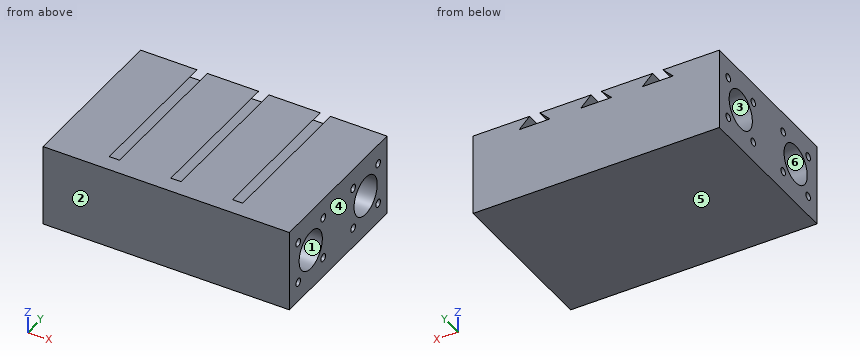
from build123d import *

# Parameters (mm, degrees)
SKETCH1_W                        = 120
SKETCH1_H                        = 80
BOSS_EXTRUDE1_DEPTH              = 40
SKETCH2_R                        = 1.85
LINEAR_BEARING_SCREW_CUTS_DEPTH  = 14
SKETCH3_R                        = 9.5
LINEAR_BEARINGS_HOLE_DEPTH       = 55
SKETCH4_R                        = 1.875
LINEAR_BEARING_SCREW_CUTS2_DEPTH = 14
LINEAR_BEARINGS_HOLE2_START      = -55
SKETCH5_R                        = 9.5
LINEAR_BEARINGS_HOLE2_DEPTH      = 55
CUT_EXTRUDE7_DEPTH               = 72


with BuildPart() as part:
    # Sketch1 → Boss-Extrude1 (new body)
    with BuildSketch(Plane.XY):
        with Locations((60, 40)):
            Rectangle(SKETCH1_W, SKETCH1_H)
    extrude(amount=BOSS_EXTRUDE1_DEPTH)

    # Sketch2 → linear-bearing-screw-cuts (cut)
    with BuildSketch(Plane.ZY):
        with Locations((30.25, 72.75)):
            Circle(SKETCH2_R)
        with Locations(Location((9.75, 72.75, 0), (0, 0, 180))):
            Circle(SKETCH2_R)
        with Locations(Location((30.25, 52.25, 0), (0, 0, 180))):
            Circle(SKETCH2_R)
        with Locations((9.75, 52.25)):
            Circle(SKETCH2_R)
        with Locations(Location((9.75, 27.75, 0), (0, 0, 180))):
            Circle(SKETCH2_R)
        with Locations((30.25, 27.75)):
            Circle(SKETCH2_R)
        with Locations(Location((30.25, 7.25, 0), (0, 0, 180))):
            Circle(SKETCH2_R)
        with Locations((9.75, 7.25)):
            Circle(SKETCH2_R)
    extrude(amount=-LINEAR_BEARING_SCREW_CUTS_DEPTH, mode=Mode.SUBTRACT)

    # Sketch3 → linear-bearings-hole (cut)
    with BuildSketch(Plane.ZY):
        with Locations((20, 62.5)):
            Circle(SKETCH3_R)
        with Locations(Location((20, 17.5, 0), (0, 0, 180))):
            Circle(SKETCH3_R)
    extrude(amount=-LINEAR_BEARINGS_HOLE_DEPTH, mode=Mode.SUBTRACT)

    # Sketch4 → linear-bearing-screw-cuts2 (cut)
    with BuildSketch(Plane(origin=(120, 0, 0), x_dir=(0, 0, -1), z_dir=(1, 0, 0))):
        with Locations((-9.75, 72.75)):
            Circle(SKETCH4_R)
        with Locations(Location((-30.25, 72.75, 0), (0, 0, 180))):
            Circle(SKETCH4_R)
        with Locations(Location((-9.75, 52.25, 0), (0, 0, 180))):
            Circle(SKETCH4_R)
        with Locations((-30.25, 52.25)):
            Circle(SKETCH4_R)
        with Locations(Location((-30.25, 27.75, 0), (0, 0, 180))):
            Circle(SKETCH4_R)
        with Locations((-9.75, 27.75)):
            Circle(SKETCH4_R)
        with Locations(Location((-9.75, 7.25, 0), (0, 0, 180))):
            Circle(SKETCH4_R)
        with Locations((-30.25, 7.25)):
            Circle(SKETCH4_R)
    extrude(amount=-LINEAR_BEARING_SCREW_CUTS2_DEPTH, mode=Mode.SUBTRACT)

    # Sketch5 → linear-bearings-hole2 (cut)
    with BuildSketch(Plane(origin=(120, 0, 0), x_dir=(0, 0, -1), z_dir=(1, 0, 0)).offset(LINEAR_BEARINGS_HOLE2_START)):
        with Locations(Location((-20, 62.5, 0), (0, 0, 180))):
            Circle(SKETCH5_R)
        with Locations((-20, 17.5)):
            Circle(SKETCH5_R)
    extrude(amount=LINEAR_BEARINGS_HOLE2_DEPTH, mode=Mode.SUBTRACT)

    # Sketch10 → Cut-Extrude7 (cut)
    with BuildSketch(Plane(origin=(0, 80, 0), x_dir=(1, 0, 0), z_dir=(0, 1, 0))):
        Polygon((92.5, -40), (97.5, -35), (82.5, -35), (87.5, -40), align=None)
        Polygon((67.5, -35), (62.5, -40), (57.5, -40), (52.5, -35), align=None)
        Polygon((37.5, -35), (32.5, -40), (27.5, -40), (22.5, -35), align=None)
    extrude(amount=-CUT_EXTRUDE7_DEPTH, mode=Mode.SUBTRACT)


solid = part.part
Work out the finished part from the listing and answer in its coordinate system (mm). Face numbers are marked on the shaded views. A direction names the side the tool comes from. Give positions to 0.01 mm unless a question says otherwise; leave off trailing zeros. Loops run counter-clockwise (first coordinate to the right, second up) from the corner with the lowest first, then second, coordinate; pieces in that order, holes last. Notation, with made-up numbers: (37, 70.25) -> (48, 70.25) arc R21 cw to (48, 90.25) -> close; hole circle Ø1 at (85.5, 75.25). An arc over 180 degrees is marked (long way). Use a Markdown table: item, result. Add a question column.
1) For a pull along Z with two mould halves and no side action, classify the marked faces 4, 5 and 6 as +Z half, -Z half, draft (parallel to the pull), parting line (faces both ways), or undercut.
2) Consider line 1 along Y through (x, z) = (115, 30); line 2 along Y through (x, z) = (17, 20.5); line 3 along Z through (x, y) = (112.25, 72.75) (3 decimals). Determine where each line is inside the solid, lowest interval first.
3) The part is cut by section C-C, the plane x = 46. Determine the outline of the cut face in (y, z).
4) Which of the six approach directions +Z, -Z, +X, -X, +Y, -Y give full straight-line access (tool end or side, diameter ignored) to the marked faces 1, 2 and 3?
5) Each of these flat-tipped pins is pushed along its axis until it touches: P1, Ø8, axis at y = 64.5, z = 22.5, coming from the +X side; P2, Ø3.5, axis at y = 72.75, z = 9.75, coming from the +X side; P3, Ø1.1, axis at y = 72, z = 9, coming from the -X side. Where does it stop, or does it pass through?
6) The part is cut by section B-B, the plane y = 17.5. Determine the outline of the cut face in (x, z), plus the area to 3 significant figures.
7) The part is cut by section A-A, the plane z = 20. Determine the outline of the cut face in (x, y).
8) The part is cut by section D-D, the plane x = 59. Determine the outline of the cut face in (y, z).
Reported:
| question | item | result |
|---|---|---|
| 1 | face 4 | draft |
| 1 | face 5 | -Z half |
| 1 | face 6 | undercut |
| 2 | line 1 | y = 0 to 5.39, 9.11 to 25.89, 29.61 to 50.39, 54.11 to 70.89, 74.61 to 80 |
| 2 | line 2 | y = 0 to 8.01, 26.99 to 53.01, 71.99 to 80 |
| 2 | line 3 | z = 0 to 7.875, 11.625 to 28.375, 32.125 to 40 |
| 3 | outline | (0, 0) -> (80, 0) -> (80, 40) -> (0, 40) -> close; hole circle Ø19 at (17.5, 20); hole circle Ø19 at (62.5, 20) |
| 4 | face 1 | +X |
| 4 | face 2 | +Z, -Z, +X, -X, -Y |
| 4 | face 3 | -X |
| 5 | P1 | stops at x = 65 |
| 5 | P2 | stops at x = 106 |
| 5 | P3 | stops at x = 14 |
| 6 | outline | (0, 0) -> (120, 0) -> (120, 10.5) -> (65, 10.5) -> (65, 29.5) -> (120, 29.5) -> (120, 40) -> (92.5, 40) -> (97.5, 35) -> (82.5, 35) -> (87.5, 40) -> (62.5, 40) -> (67.5, 35) -> (52.5, 35) -> (57.5, 40) -> (32.5, 40) -> (37.5, 35) -> (22.5, 35) -> (27.5, 40) -> (0, 40) -> (0, 29.5) -> (55, 29.5) -> (55, 10.5) -> (0, 10.5) -> close |
| 6 | area | 2,560 mm^2 |
| 7 | outline | (0, 0) -> (120, 0) -> (120, 8) -> (65, 8) -> (65, 27) -> (120, 27) -> (120, 53) -> (65, 53) -> (65, 72) -> (120, 72) -> (120, 80) -> (0, 80) -> (0, 72) -> (55, 72) -> (55, 53) -> (0, 53) -> (0, 27) -> (55, 27) -> (55, 8) -> (0, 8) -> close |
| 8 | outline | (0, 0) -> (80, 0) -> (80, 35) -> (8, 35) -> (8, 40) -> (0, 40) -> close |
